from build123d import *

# Parameters (mm, degrees)
SKETCH1_W           = 43
SKETCH1_H           = 32
SKETCH1_W_2         = 37
SKETCH1_H_2         = 26
BOSS_EXTRUDE1_DEPTH = 10
SKETCH2_W           = 13
SKETCH2_H           = 3
BOSS_EXTRUDE2_DEPTH = 15
CUT_EXTRUDE1_REACH  = 34
SKETCH3_R           = 1.905
SKETCH4_W           = 43
SKETCH4_H           = 32
BOSS_EXTRUDE3_DEPTH = 2
CUT_EXTRUDE2_REACH  = 29
SKETCH5_R           = 10
BOSS_EXTRUDE4_START = -5
SKETCH14_R          = 2.75
BOSS_EXTRUDE4_DEPTH = 25
SKETCH16_R          = 1.75
CUT_EXTRUDE3_DEPTH  = 30
SKETCH17_R          = 2.5
CUT_EXTRUDE4_DEPTH  = 10


with BuildPart() as part:
    # Sketch1 → Boss-Extrude1 (new body)
    with BuildSketch(Plane(origin=(0, 0, 0), x_dir=(1, 0, 0), z_dir=(0, 1, 0))):
        with Locations((18.5, 13)):
            Rectangle(SKETCH1_W, SKETCH1_H)
        with Locations((18.5, 13)):
            Rectangle(SKETCH1_W_2, SKETCH1_H_2, mode=Mode.SUBTRACT)
    extrude(amount=BOSS_EXTRUDE1_DEPTH)

    # Sketch2 → Boss-Extrude2 (add)
    with BuildSketch(Plane(origin=(0, 10, 0), x_dir=(1, 0, 0), z_dir=(0, 1, 0))):
        with Locations((18.5, 27.5)):
            Rectangle(SKETCH2_W, SKETCH2_H)
    extrude(amount=BOSS_EXTRUDE2_DEPTH)

    # Sketch3 → Cut-Extrude1 (cut, up to next)
    with BuildSketch(Plane(origin=(0, 0, -29), x_dir=(-1, 0, 0), z_dir=(0, 0, -1)), mode=Mode.PRIVATE) as cut_extrude1_sk1:
        with Locations((-18.5, 21)):
            Circle(SKETCH3_R)
    cut_extrude1_tool1 = extrude(cut_extrude1_sk1.sketch, amount=-CUT_EXTRUDE1_REACH, mode=Mode.PRIVATE) & part.part
    add(cut_extrude1_tool1.solids().sort_by_distance((18.5, 21, -29))[0], mode=Mode.SUBTRACT)

    # Sketch4 → Boss-Extrude3 (add)
    with BuildSketch(Plane.XZ):
        with Locations((18.5, -13)):
            Rectangle(SKETCH4_W, SKETCH4_H)
    extrude(amount=BOSS_EXTRUDE3_DEPTH)

    # Sketch5 → Cut-Extrude2 (cut, up to next)
    with BuildSketch(Plane.XZ.offset(2), mode=Mode.PRIVATE) as cut_extrude2_sk1:
        with Locations((18.5, -13)):
            Circle(SKETCH5_R)
    cut_extrude2_tool1 = extrude(cut_extrude2_sk1.sketch, amount=-CUT_EXTRUDE2_REACH, mode=Mode.PRIVATE) & part.part
    add(cut_extrude2_tool1.solids().sort_by_distance((18.5, -2, -13))[0], mode=Mode.SUBTRACT)

    # Sketch9 → Revolve1 (revolve)
    with BuildSketch(Plane.XY.offset(-13)):
        Polygon((28.5, 0), (21.5, -33.75), (22.5, -33.75), (33.5, 0), align=None)
    revolve(axis=Axis((18.5, -2, -13), (0, -1, 0)))

    # Sketch14 → Boss-Extrude4 (add)
    with BuildSketch(Plane(origin=(18.5, -13.221888935, -28.050276014), x_dir=(-1, 0, 0), z_dir=(0, -0.784602856, 0.619998676)).offset(BOSS_EXTRUDE4_START)):
        with Locations((0.305660396, 0)):
            Circle(SKETCH14_R)
    extrude(amount=BOSS_EXTRUDE4_DEPTH)

    # Sketch16 → Cut-Extrude3 (cut)
    with BuildSketch(Plane(origin=(0, 9.428731153, -7.45064945), x_dir=(1, 0, 0), z_dir=(0, 0.784602856, -0.619998676))):
        with Locations((18.194339604, 30.205880304)):
            Circle(SKETCH16_R)
    extrude(amount=-CUT_EXTRUDE3_DEPTH, mode=Mode.SUBTRACT)

    # Sketch17 → Cut-Extrude4 (cut)
    with BuildSketch(Plane.XZ.offset(33.75)):
        with Locations((18.5, -13)):
            Circle(SKETCH17_R)
    extrude(amount=-CUT_EXTRUDE4_DEPTH, mode=Mode.SUBTRACT)


solid = part.part
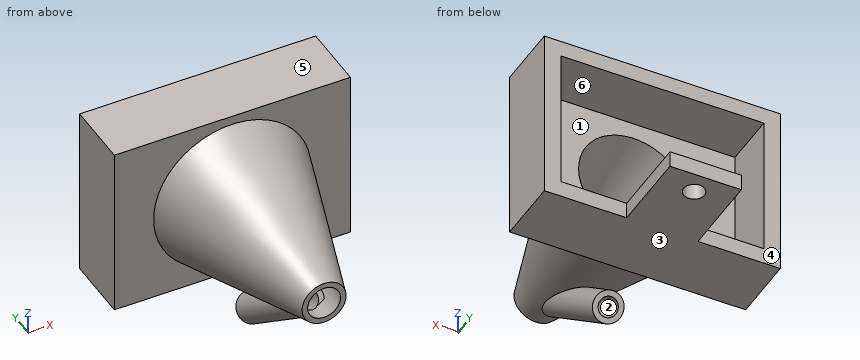
Geometry: final body of the model. Coordinates: model frame, mm. Face numbers are marked on the shaded views. A direction names the side the tool comes from. Give positions to 0.01 mm unless a question says otherwise; leave off trailing zeros. Loops run counter-clockwise (first coordinate to the right, second up) from the corner with the lowest first, then second, coordinate; pieces in that order, holes last. Notation, with made-up numbers: M 26.25,40 L 48.25,40 A28 ccw 48.25,68 Z; hole C 46.5,2.25 d10. An arc over 180 degrees is marked long. Put each result on its own line as item: value. Start each with the question number.
1) Cut plane A-A (z = -13). Output: boundary loops of the cut face in (x, y).
2) Cut plane D-D (x = 35). Output: boundary loops of the cut face in (y, z), then the cut area to 3 significant figures.
3) Access query for the marked faces 1, 2 and 3. Directions: +Z, -Z, +X, -X, +Y, -Y. A direction counts if a zero-diameter tool reaches every point of the face in a straight line with its end or side. Return the directions, or none.
4) Cut plane B-B (y = 21). Output: boundary loops of the cut face in (x, z) (3 decimals), then the cut area to 3 significant figures.
5) Contact query for flat-ended pins moving along their axis: pin 1 (4 mm diameter, centred on x = 33, z = -5.5, fed in from +Y); pin 2 (8 mm diameter, centred on y = 16, z = -17.5, fed in from +X); pin 3 (2 mm diameter, centred on y = -10.5, z = -21, fed in from -X); pin 4 (0.9 mm diameter, centred on y = 17, z = -28, fed in from +X). Output: stop coordinate, or through.
6) Pull-direction query (Z, two-part tool) for the marked faces 4, 5 and 6; classes: pulls with the +Z half, pulls with the -Z half, needs draft (parallel to the pull), parting line crosses it, or undercut.
7) Cut plane C-C (x = 18.5). Give the number of separate pieces and of enclosed holes in the cut face, then the cut area to 3 significant figures.
8) Ray query, line 1 along Z through (x, y) = (2.5, 4.5); line 2 along Y through (x, z) = (18.5, -28.2) (3 decimals); line 3 along Y through (x, z) = (18.5, -27.7) (3 decimals). Return the intervals inside material, ascending.
Verdict:
1. outline: M -3,-2 L 4.15,-2 L 14.5,-33.75 L 15.5,-33.75 L 8.5,0 L 0,0 L 0,10 L -3,10 Z; M 21.5,-33.75 L 22.5,-33.75 L 32.85,-2 L 40,-2 L 40,10 L 37,10 L 37,0 L 28.5,0 Z
2. outline: M -2,-29 L 10,-29 L 10,-26 L 0,-26 L 0,0 L 10,0 L 10,3 L -2,3 Z
2. area: 124 mm2
3. face 1: +Y
3. face 2: none
3. face 3: -Z, +X, -X, +Y
4. outline: M 12,-29 L 16.595,-29 L 16.595,-26 L 12,-26 Z; M 20.405,-29 L 25,-29 L 25,-26 L 20.405,-26 Z
4. area: 27.6 mm2
5. pin 1: y = 0
5. pin 2: through
5. pin 3: x = 9.17
5. pin 4: x = 25
6. face 4: needs draft
6. face 5: pulls with the +Z half
6. face 6: undercut
7. separate pieces: 4
7. enclosed holes: 0
7. area: 323 mm2
8. line 1: -29 to -26, 0 to 3
8. line 2: -17.44 to -15.812, -10.253 to -8.624, -2 to 19.095, 22.905 to 25
8. line 3: -18.073 to -16.444, -10.886 to -9.257, -2 to 19.095, 22.905 to 25
